For this review, take the finished solid that the model builds, in its own axes (mm). Round coordinates to 2 decimals unless told otherwise and drop trailing zeros. Write each loop counter-clockwise with the first axis right and the second up, starting at its lowest first coordinate (ties: lowest second). Pieces come first, ordered by that corner, then holes. Notation, with made-up numbers: (-15.5, 36) -> (28.5, 36) arc R21 ccw to (28.5, 57) -> close; hole circle Ø4 at (-4, 87). An arc over 180 degrees is marked (long way). Write each question's results on one line, items separated by ' | '. Start each with the question number.
Item 1: Add section C-C (z = 48.5). State the section outline as (x, y) points, plus the area to 3 significant figures.
Item 2: To check wall thickness, follow line 1 along Y through (x, z) = (0, 211.75) (3 decimals); line 2 along Z through (x, y) = (0, -4.25); line 3 along Z through (x, y) = (0, 1). State the ranges of each line that lie inside material, in increasing order.
Item 3: Clearance check with flat-ended pins moving along their axes: pin 1 (12 mm diameter, centred on y = -9, z = 190, fed in from -X); pin 2 (5 mm diameter, centred on y = -3, z = 92, fed in from -X); pin 3 (1.5 mm diameter, centred on x = 5, z = 142, fed in from -Y). State where each tip first meets the part, or that it passes through.
Item 4: Add section D-D (z = 196.85). State the section outline as (x, y) points, plus the area to 3 significant figures.
Item 5: Add section A-A (x = 0). State the section outline as (y, z) points (1 decimal).
from build123d import *

# Parameters (mm, degrees)
F0_R          = 12.7
F1_DEPTH      = 215.9
F2_SIZE2      = 5.08
F2_SIZE       = 17.78
F3_R          = 4.7625
F4_DEPTH      = 25.4
F4_DEPTH_BACK = 25.4
F5_R          = 3.175
F6_DEPTH      = 12.7


with BuildPart() as f1:
    # F0 (on Top) → F1 (new body)
    with BuildSketch(Plane.XY):
        Circle(F0_R)
    extrude(amount=F1_DEPTH)

    # F2
    f2_edges = [f1.edges().sort_by_distance(p)[0] for p in [
        (-12.7, 0, 0),
    ]]
    chamfer(f2_edges, length=F2_SIZE, length2=F2_SIZE2)

    # F3 (on Front) → F4 (cut, two sides)
    with BuildSketch(Plane.XZ) as f4_sk:
        with Locations((0, 196.85)):
            Circle(F3_R)
    extrude(amount=F4_DEPTH, mode=Mode.SUBTRACT)
    extrude(f4_sk.sketch, amount=-F4_DEPTH_BACK, mode=Mode.SUBTRACT)

    # F5 (on face) → F6 (cut)
    with BuildSketch(Plane.XY.offset(215.9)):
        Circle(F5_R)
    extrude(amount=-F6_DEPTH, mode=Mode.SUBTRACT)


solid = f1.part
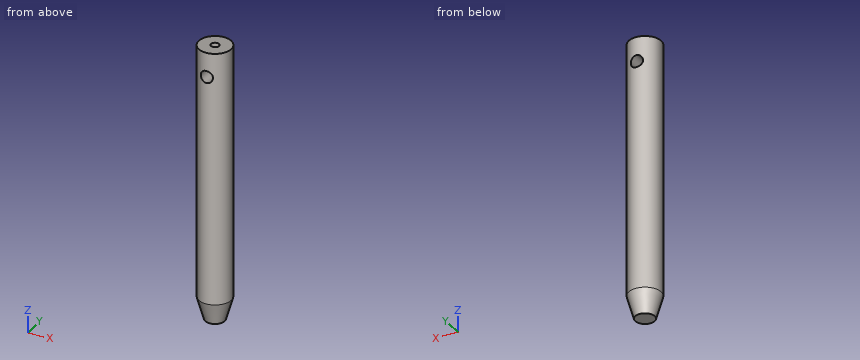
Responses:
1) outline: circle Ø25.4 at (0, 0) | area: 507 mm^2
2) line 1: y = -12.7 to -3.175, 3.175 to 12.7 | line 2: z = 0 to 192.09, 201.61 to 215.9 | line 3: z = 0 to 192.09, 201.61 to 203.2
3) pin 1: stops at x = -12.34 | pin 2: stops at x = -12.69 | pin 3: stops at y = -11.97
4) outline: (-4.76, -11.77) -> (-4.76, 11.77) arc R12.7 ccw to start; (4.76, -11.77) arc R12.7 ccw to (4.76, 11.77) -> close | area: 271 mm^2
5) outline: (-12.7, 17.8) -> (-7.6, 0) -> (7.6, 0) -> (12.7, 17.8) -> (12.7, 192.1) -> (-12.7, 192.1) -> close; (-12.7, 201.6) -> (12.7, 201.6) -> (12.7, 215.9) -> (3.2, 215.9) -> (3.2, 203.2) -> (-3.2, 203.2) -> (-3.2, 215.9) -> (-12.7, 215.9) -> close
